Could you check a few things on this drawing? It's one solid part, dimensions in mm from its lowest x, y, z. A direction names the side the tool comes from. Coordinates: 2 decimals unless noted, no trailing zeros. Write each loop counter-clockwise with the first axis right and the second up, starting at its lowest first coordinate (ties: lowest second). Pieces come first, ordered by that corner, then holes. Notation, with made-up numbers: (-8, 39.25) - (-1, 39.25) arc R8 cw to (-1, 53.25) - close; hole circle Ø2 at (-2.75, 82.5). An arc over 180 degrees is marked (long way). Write item = value, one per line. Start each with the question number.
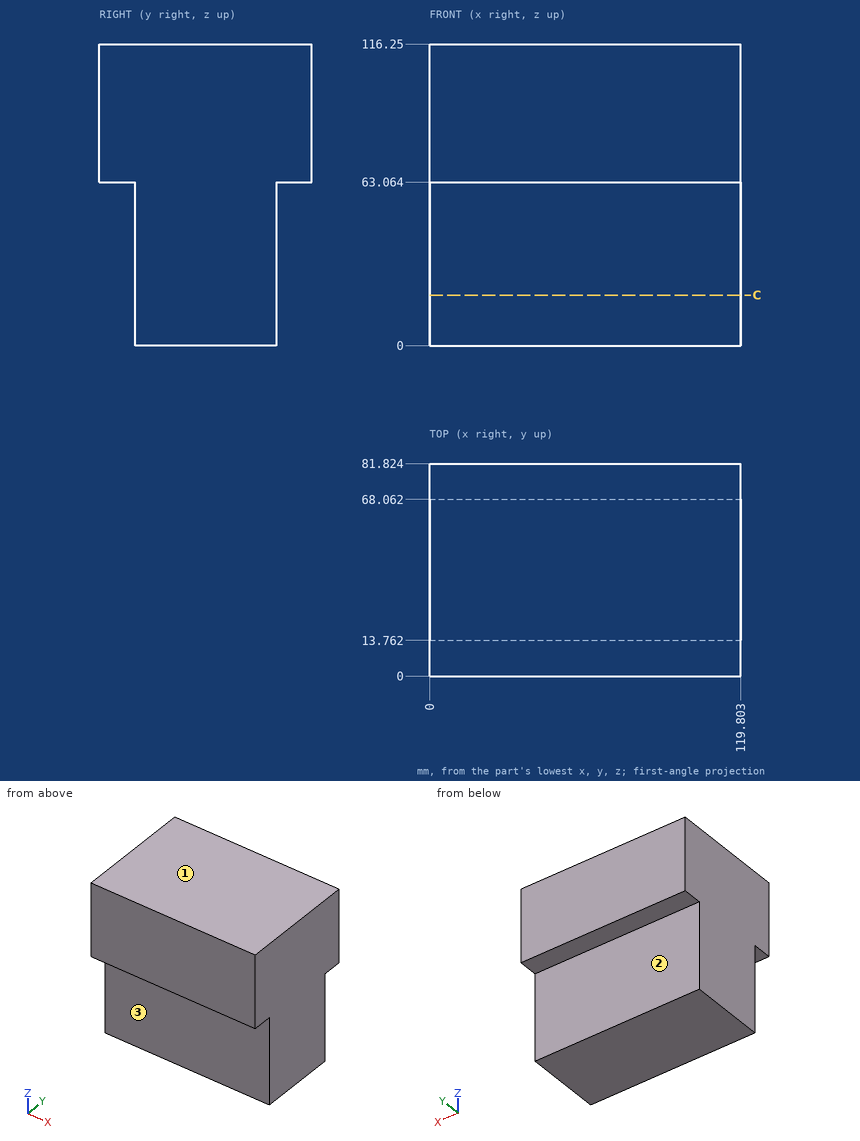
1) If I drill on probe 1 along Y at (x, z) = (13.5, 50), over which ranges is the centre line in solid material (lowest first)? Write a range as [from, to].
2) Suppose I cut it at C-C on z = 19.5. Please give me the cut outline in (x, y), plus the area to 3 significant figures.
3) For P1, Ø1.5, axis at x = 54.5, z = 42, coming from the -Y side; P2, Ø4, axis at x = 22.5, z = 29.5, coming from the +Y side; P3, Ø15, axis at x = 44, y = 6, coming from the -Z side, each with a flat end and sliding along its axis, tell me the tip position at first contact or that it passes through.
4) Which directions (+Z, -Z, +X, -X, +Y, -Y) give clear straight access to the entire face, cutting with the end or side of a thin tool? Please do the marked faces 1, 2 and 3.
Reply:
q1.probe_1 = [13.76, 68.06]
q2.outline = (0, 13.76) - (119.8, 13.76) - (119.8, 68.06) - (0, 68.06) - close
q2.area = 6,510 mm^2
q3.P1 = 13.76
q3.P2 = 68.06
q3.P3 = 63.06
q4.face_1 = +Z, +X, -X, +Y, -Y
q4.face_2 = -Z, +X, -X, +Y
q4.face_3 = -Z, +X, -X, -Y
